For this review, take the finished solid that the model builds, in its own axes (mm). A direction names the side the tool comes from. Give positions to 0.01 mm unless a question says otherwise; leave off trailing zeros. Loops run counter-clockwise (first coordinate to the right, second up) from the corner with the lowest first, then second, coordinate; pieces in that order, holes last. Notation, with made-up numbers: (52, 7) -> (76, 7) arc R16 cw to (76, 32) -> close; hole circle Ø9 at (17, 78.5). An arc over 180 degrees is marked (long way). Write each question's results on one line, items separated by ' | '. Start each with the question number.
```python
from build123d import *

# Parameters (mm, degrees)
OBR_T1_ANGLE                = 180
WYTNIJ_WYCI_GNI_CIE1_DEPTH  = 172.464281995
WYTNIJ_WYCI_GNI_CIE2_DEPTH  = 147.710676959
SFAZOWANIE1_SIZE            = 5
SKORUPA1_T                  = -2
DODANIE_WYCI_GNI_CIE1_DEPTH = 2


with BuildPart() as part:
    # Szkic1 → Obrót1 (revolve)
    with BuildSketch(Plane(origin=(0, 0, 0), x_dir=(0, 0, -1), z_dir=(1, 0, 0))):
        with BuildLine():
            Line((0, -55), (0, 55))
            Line((0, 55), (-75, 55))
            ThreePointArc((-75, 55), (-93.005376189, 0), (-75, -55))
            Line((-75, -55), (0, -55))
        make_face()
    revolve(axis=Axis((0, -55, 0), (0, 1, 0)), revolution_arc=OBR_T1_ANGLE)

    # Szkic2 → Wytnij-wyciągnięcie1 (cut, through all)
    with BuildSketch(Plane.XZ.offset(55)):
        Polygon((0, 0), (0, 40), (12.287280664, 48.603646545), (12.287280664, 99.487677337), (-26.065901524, 99.487677337), (-26.065901524, -104.75854766), (87.353699516, -104.75854766), (87.353699516, -51.998360457), (17.67766953, 17.67766953), align=None)
    extrude(amount=-WYTNIJ_WYCI_GNI_CIE1_DEPTH, mode=Mode.SUBTRACT)

    # Szkic3 → Wytnij-wyciągnięcie2 (cut, through all)
    with BuildSketch(Plane(origin=(100, 0, 0), x_dir=(0, 0, -1), z_dir=(1, 0, 0))):
        Polygon((-60, -15), (-60, 15), (45.666627767, 30), (45.666627767, -30), align=None)
    extrude(amount=-WYTNIJ_WYCI_GNI_CIE2_DEPTH, mode=Mode.SUBTRACT)

    # Sfazowanie1
    # the kernel refuses this chamfer: 5, 4.450979534 mm, written as the material it takes off along each edge
    with BuildSketch(Plane(origin=(12.287280664, 0, 0), x_dir=(0, 0.7023997796774998, 0.7117826560889214), z_dir=(0, 0.7117826560889214, -0.7023997796774998))) as sfazowanie1_piece_1:
        with BuildLine():
            Line((92.190144451 - SFAZOWANIE1_SIZE, 0), (91.510568486, 4.320424035))
            ThreePointArc((91.510568486, 4.320424035), (91.866596239, 2.222319448), (92.190144451, 0))
            Line((92.190144451, 0), (92.190144451 - SFAZOWANIE1_SIZE, 0))
        make_face()
    revolve(axis=Axis((12.287280664, 0, 0), (1, 0, 0)), revolution_arc=89.239714317, mode=Mode.SUBTRACT)

    # Skorupa1
    skorupa1_openings = [part.faces().sort_by_distance(p)[0] for p in [
        (0, 37.799975499, 20.551470825),
        (44.318791783, 39.564539913, -8.963452724),
        (12.287280664, 0, 66.554150501),
        (8.951756718, 38.623299359, 8.951756718),
        (6.176749303, 36.112578818, 44.325006424),
        (8.951756718, -38.623299359, 8.951756718),
        (44.318791783, -39.564539913, -8.963452724),
        (6.176749303, -36.112578818, 44.325006424),
        (0, -37.799975499, 20.551470825),
        (41.411625019, 0, 60),
        (50.400096072, -20.67683416, 20.009871862),
        (50.400096072, 20.67683416, 20.009871862),
    ]]
    offset(amount=SKORUPA1_T, openings=skorupa1_openings)

    # Szkic4 → Dodanie-wyciągnięcie1 (add)
    with BuildSketch(Plane.XZ.offset(55)):
        Polygon((0, 40), (0, 51.81910108), (12.287280664, 67.654425497), (12.287280664, 48.603646545), align=None)
    dodanie_wyci_gni_cie1 = extrude(amount=-DODANIE_WYCI_GNI_CIE1_DEPTH)

    # Lustro1: Dodanie-wyciągnięcie1 across plane
    add(dodanie_wyci_gni_cie1.mirror(Plane.ZX))


solid = part.part
```
1. We need section B-B (x = 29.5). Write out the cut boundary in (y, z).
2. For pin 1 Ø12 at (x, z) = (64, 65.5) entering from +Y; pin 2 Ø12 at (y, z) = (21.5, 53.5) entering from -X; pin 3 Ø3 at (y, z) = (23, 13) entering from -X; pin 4 Ø12 at (x, z) = (40, -16) entering from -Y, all flat-tipped, find the tip position at first contact; note any pin that passes through.
3. Wall thickness on L1, parallel to Y at x = 32, z = 18.5; L2, parallel to Y at x = 45, z = 70.5; L3, parallel to Z at x = 58, y = 6: over which ranges is each line inside the solid? List them lowest first.
4. Draft analysis for pull direction X (two halves, no side actions). For faces 1 (the flat face through (12.287, 4, 85)), 2 (the flat face through (87.942, 22.215, 9.171)), 3 (the flat face through (9, -54, 9)), 4 (the conical face through (12.6, 0.81, 84.67)), state which applies: released by +X, released by -X, zero draft, split by the parting line, or undercut.
5. We need section A-A (z = -22.5). Write out the cut boundary in (x, y), plus the area to 3 significant figures.
6. We need section D-D (x = 65). Write out the cut boundary in (y, z), plus the area to 3 significant figures.
7. We need section C-C (z = 43). Write out the cut boundary in (x, y).
8. Machinability: for faces 5 (the flat face through (6.06, 54.01, 59.63)), 6 (the flat face through (9, 54, 9)), 7 (the flat face through (87.942, -21.746, 12.477)), which of the approach directions +Z, -Z, +X, -X, +Y, -Y give a long, thin tool a straight path to every point of the face, cutting with its end or side? Answer none if there is none.
Response:
1) outline: (-55, 5.86) -> (-53, 5.86) -> (-53, 67.84) arc R86.09 cw to (53, 67.84) -> (53, 5.86) -> (55, 5.86) -> (55, 68.95) arc R88.2 ccw to (-55, 68.95) -> close
2) pin 1: stops at y = 36.42 | pin 2: stops at x = 65.04 | pin 3: stops at x = 86.62 | pin 4: passes through
3) L1: y = -55 to -53, 53 to 55 | L2: y = -40.68 to -35.87, 35.87 to 40.68 | L3: z = 69.87 to 72.46
4) face 1: released by -X | face 2: zero draft | face 3: undercut | face 4: undercut
5) outline: (57.86, -55) -> (71.55, -55) arc R90.24 ccw to (86.2, -26.71) -> (84.04, -26.71) arc R88.18 cw to (70.48, -53) -> (57.86, -53) -> close; (57.86, 53) -> (70.48, 53) arc R88.18 cw to (84.04, 26.71) -> (86.2, 26.71) arc R90.24 ccw to (71.55, 55) -> (57.86, 55) -> close | area: 180 mm2
6) outline: (-55, -29.64) -> (-53, -29.64) -> (-53, 35.33) arc R63.69 cw to (53, 35.33) -> (53, -29.64) -> (55, -29.64) -> (55, 37.42) arc R66.52 ccw to (-55, 37.42) -> close | area: 624 mm2
7) outline: (0, -55) -> (61.45, -55) arc R82.47 ccw to (80.61, -17.41) -> (78.29, -17.41) arc R80.21 cw to (60.2, -53) -> (0, -53) -> close; (0, 53) -> (60.2, 53) arc R80.21 cw to (78.29, 17.41) -> (80.61, 17.41) arc R82.47 ccw to (61.45, 55) -> (0, 55) -> close
8) face 5: +Z, -X, +Y, -Y | face 6: -Z, +Y, -Y | face 7: -Z, +X, -X
